from build123d import *

# Parameters (mm, degrees)
SKETCH1_W                      = 152.421392062
SKETCH1_H                      = 12
BOSS_EXTRUDE1_DEPTH            = 3.5
CUT_EXTRUDE1_DEPTH             = 3.1
CUT_EXTRUDE2_DEPTH             = 3.1
CUT_EXTRUDE3_DEPTH             = 3.1
F_3_5_3_5_DIAMETER_HOLE1_D     = 3.5
F_3_5_3_5_DIAMETER_HOLE1_DEPTH = 0.4
FILLET1_R                      = 0.150000007


with BuildPart() as part:
    # Sketch1 → Boss-Extrude1 (new body)
    with BuildSketch(Plane(origin=(0, 0, 0), x_dir=(-1, 0, 0), z_dir=(0, 0, -1))):
        with Locations((15.639629555, 0)):
            Rectangle(SKETCH1_W, SKETCH1_H)
    extrude(amount=-BOSS_EXTRUDE1_DEPTH)

    # Sketch2 → Cut-Extrude1 (cut)
    with BuildSketch(Plane(origin=(0, 0, 0), x_dir=(-1, 0, 0), z_dir=(0, 0, -1))):
        Polygon((17.674321891, -2.900007341), (19.348637675, -7.335e-06), (17.674319972, 2.899992671), (14.325688404, 2.899992671), (12.651373579, -7.889e-06), (14.325690323, -2.900007341), align=None)
    extrude(amount=-CUT_EXTRUDE1_DEPTH, mode=Mode.SUBTRACT)

    # Sketch3 → Cut-Extrude2 (cut)
    with BuildSketch(Plane(origin=(0, 0, 0), x_dir=(-1, 0, 0), z_dir=(0, 0, -1))):
        Polygon((-57.919692896, -7.889e-06), (-56.245376153, -2.900007341), (-52.896744585, -2.900007341), (-51.2224288, -7.335e-06), (-52.896746503, 2.899992671), (-56.245378072, 2.899992671), align=None)
    extrude(amount=-CUT_EXTRUDE2_DEPTH, mode=Mode.SUBTRACT)

    # Sketch4 → Cut-Extrude3 (cut)
    with BuildSketch(Plane(origin=(0, 0, 0), x_dir=(-1, 0, 0), z_dir=(0, 0, -1))):
        Polygon((82.501699166, -7.889e-06), (84.176015909, -2.900007341), (87.524647477, -2.900007341), (89.198963262, -7.335e-06), (87.524645559, 2.899992671), (84.17601399, 2.899992671), align=None)
    extrude(amount=-CUT_EXTRUDE3_DEPTH, mode=Mode.SUBTRACT)

    # Ø3.5 (3.5) Diameter Hole1
    with Locations(Plane(origin=(0, 0, 3.1), x_dir=(-1, 0, 0), z_dir=(0, 0, -1))):
        with Locations((-54.571061328, 6.781e-06), (85.850330734, 6.781e-06), (16, 0)):
            Hole(F_3_5_3_5_DIAMETER_HOLE1_D / 2, depth=F_3_5_3_5_DIAMETER_HOLE1_DEPTH)

    # Fillet1
    fillet1_edges = [part.edges().sort_by_distance(p)[0] for p in [
        (-17.674321891, -2.900007341, 1.55),
        (-14.325690323, -2.900007341, 1.55),
        (-12.651373579, -7.889e-06, 1.55),
        (-14.325688404, 2.899992671, 1.55),
        (-17.674319972, 2.899992671, 1.55),
        (-19.348637675, -7.335e-06, 1.55),
        (57.919692896, -7.889e-06, 1.55),
        (56.245378072, 2.899992671, 1.55),
        (52.896746503, 2.899992671, 1.55),
        (51.2224288, -7.335e-06, 1.55),
        (52.896744585, -2.900007341, 1.55),
        (56.245376153, -2.900007341, 1.55),
        (-82.501699166, -7.889e-06, 1.55),
        (-84.17601399, 2.899992671, 1.55),
        (-87.524645559, 2.899992671, 1.55),
        (-89.198963262, -7.335e-06, 1.55),
        (-87.524647477, -2.900007341, 1.55),
        (-84.176015909, -2.900007341, 1.55),
    ]]
    fillet(fillet1_edges, radius=FILLET1_R)


solid = part.part
Part model, mm, in its own coordinate system. A direction names the side the tool comes from. Give positions to 0.01 mm unless a question says otherwise; leave off trailing zeros. Loops run counter-clockwise (first coordinate to the right, second up) from the corner with the lowest first, then second, coordinate; pieces in that order, holes last. Notation, with made-up numbers: (63, -25) -> (113, -25) arc R24 cw to (113, 4) -> close; hole circle Ø7 at (84.25, 72). An arc over 180 degrees is marked (long way). Write each question's results on one line, items separated by ' | '. Start each with the question number.
Q1. Which spindle directions (+Z, -Z, +X, -X, +Y, -Y) get a long thin tool onto all of the face, cutting with end or side? Do faces 5 (the face through (-15, 4, 0)), 6 (the face through (53.1, 1.3, 3.1)). Say none if no direction does.
Q2. Band-saw the part on A-A on x = -16. List the corners of the cut face in (y, z), plus the area to 3 significant figures.
Q3. Pull direction X, two halves, no side cores. Call faces 1 (the face through (57.094, -1.431, 1.528)), 2 (the face through (60.571, 0, 2)), 3 (the face through (-14.6, 1.4, 3.5)), 4 (the face through (-91.85, 0, 2)): +X half, -X half, draft (parallel to the pull), parting line (faces both ways), or undercut.
Q4. Pin check, flat tips, straight feed: P1, Ø4, axis at x = -85.85, y = 0, coming from the -Z side; P2, Ø4.5, axis at x = 56, y = -1, coming from the -Z side; P3, Ø3, axis at x = 54.57, y = 0, coming from the -Z side. Stop position of each tip, or through.
Q5. Wall check: L1, parallel to X at y = -2.75, z = 0.8; L2, parallel to X at y = -2.25, z = 0.6; L3, parallel to Y at x = -16, z = 3.45. Give the ranges that are in metal, low to high.
Q6. Band-saw the part on B-B on z = 0.9. Count the separate pieces of the cut face and the enclosed holes in it, plus the area to 3 significant figures.
Results are:
1) face 5: -Z, +X, -X, +Y, -Y | face 6: -Z
2) outline: (-6, 0) -> (-2.9, 0) -> (-2.9, 3.1) -> (-1.75, 3.1) -> (-1.75, 3.5) -> (-6, 3.5) -> close; (1.75, 3.1) -> (2.9, 3.1) -> (2.9, 0) -> (6, 0) -> (6, 3.5) -> (1.75, 3.5) -> close | area: 22.6 mm²
3) face 1: undercut | face 2: +X half | face 3: draft | face 4: -X half
4) P1: stops at z = 3.1 | P2: stops at z = 0 | P3: passes through
5) L1: x = -91.85 to -87.61, -84.09 to -17.76, -14.24 to 52.81, 56.33 to 60.57 | L2: x = -91.85 to -87.9, -83.8 to -18.05, -13.95 to 52.52, 56.62 to 60.57 | L3: y = -6 to -1.75, 1.75 to 6
6) separate pieces: 1 | enclosed holes: 3 | area: 1,740 mm²
